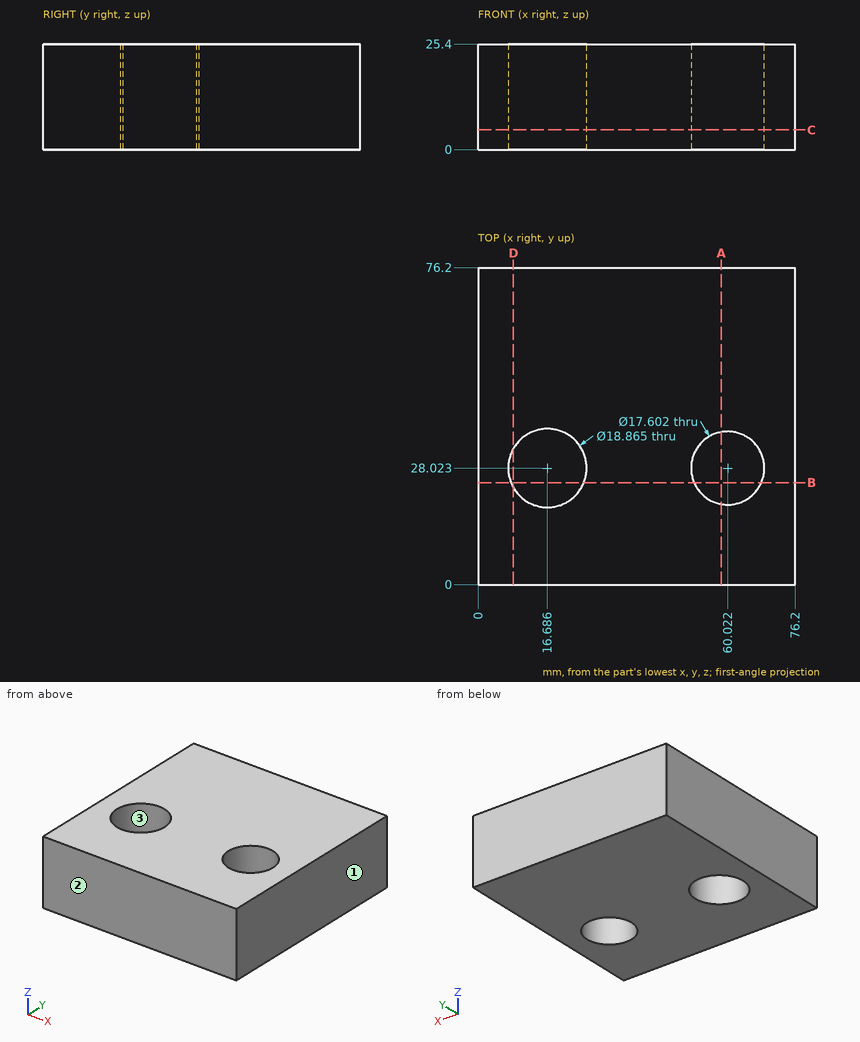
Job drawing, mm, ordinate dimensions from the low corner. One solid piece. Coordinates: 2 decimals unless noted, no trailing zeros. Order: outer loops, then holes, each group sorted by start corner. A loop starts at its lowest first (then second) coordinate and runs counter-clockwise, first axis right, second up. Notation, with made-up numbers: (45, 74.25) - (55, 74.25) arc R21 cw to (55, 95.25) - close; hole circle Ø7 at (66.25, 31.5). An arc over 180 degrees is marked (long way). Write each question's results on one line, items separated by ' | '. Start each with the question number.
Item 1: Band-saw the part on C-C on z = 4.75. Write the cut outline in (x, y) (1 decimal), and give its area (3 significant figures).
Item 2: Band-saw the part on A-A on x = 58.5. Write the cut outline in (y, z) (1 decimal).
Item 3: Band-saw the part on B-B on y = 24.5. Write the cut outline in (x, z).
Item 4: Wall check: probe 1 along X at (y, z) = (34, 15.5) (1 decimal); probe 2 along X at (y, z) = (27, 23.5); probe 3 along Y at (x, z) = (17, 9.75). Give the ranges that are in metal, low to high. Write a range as [from, to].
Item 5: Mould opens along Y. For the marked faces 1, 2 and 3 say: released by +Y, released by -Y, zero draft, split by the parting line, or undercut.
Item 6: Band-saw the part on D-D on x = 8.5. Write the cut outline in (y, z).
Numbers:
1) outline: (0, 0) - (76.2, 0) - (76.2, 76.2) - (0, 76.2) - close; hole circle Ø18.9 at (16.7, 28); hole circle Ø17.6 at (60, 28) | area: 5,280 mm^2
2) outline: (0, 0) - (19.4, 0) - (19.4, 25.4) - (0, 25.4) - close; (36.7, 0) - (76.2, 0) - (76.2, 25.4) - (36.7, 25.4) - close
3) outline: (0, 0) - (7.94, 0) - (7.94, 25.4) - (0, 25.4) - close; (25.44, 0) - (51.96, 0) - (51.96, 25.4) - (25.44, 25.4) - close; (68.09, 0) - (76.2, 0) - (76.2, 25.4) - (68.09, 25.4) - close
4) probe 1: [0, 9.4], [24, 53.6], [66.5, 76.2] | probe 2: [0, 7.31], [26.06, 51.28], [68.76, 76.2] | probe 3: [0, 18.6], [37.45, 76.2]
5) face 1: zero draft | face 2: released by -Y | face 3: undercut
6) outline: (0, 0) - (23.34, 0) - (23.34, 25.4) - (0, 25.4) - close; (32.71, 0) - (76.2, 0) - (76.2, 25.4) - (32.71, 25.4) - close
